The drawing under review shows one solid part. Ordinate dimensions are in mm from its lowest x, y, z. Give positions to 0.01 mm unless a question says otherwise; leave off trailing zeros. Loops run counter-clockwise (first coordinate to the right, second up) from the corner with the lowest first, then second, coordinate; pieces in that order, holes last. Notation, with made-up numbers: M -35.5,58 L -21.5,58 A29 cw -21.5,88 Z; hole C 48.25,49 d3. An arc over 180 degrees is marked long. One line per item, written item: value. Start each with the question number.
Q1. To check wall thickness, follow line 1 along Y through (x, z) = (40.5, 39); line 2 along Y through (x, z) = (42, 30.5) (1 decimal); line 3 along Z through (x, y) = (12.5, 26). State the ranges of each line that lie inside material, in increasing order. Write a range as from..to.
Q2. Mouldability with a two-part tool opening along X and no side actions: class the marked faces 1, 2 and 3 as released by +X, released by -X, zero draft, split by the parting line, or undercut.
Q3. We need section A-A on z = 49. Write out the cut boundary in (x, y) (1 decimal).
Q4. For pin 1 (3 mm diameter, centred on x = 34, z = 46, fed in from +Y); pin 2 (1 mm diameter, centred on x = 44, y = 45.5, fed in from +Z); pin 3 (3 mm diameter, centred on x = 37, z = 49, fed in from -Y) (1 decimal); pin 4 (10 mm diameter, centred on x = 60.5, y = 19, fed in from -Z), all flat-tipped, find the tip position at first contact; note any pin that passes through.
Q5. We need section C-C on y = 62. Write out the cut boundary in (x, z).
Q6. We need section B-B on x = 32. Write out the cut boundary in (y, z), plus the area to 3 significant figures.
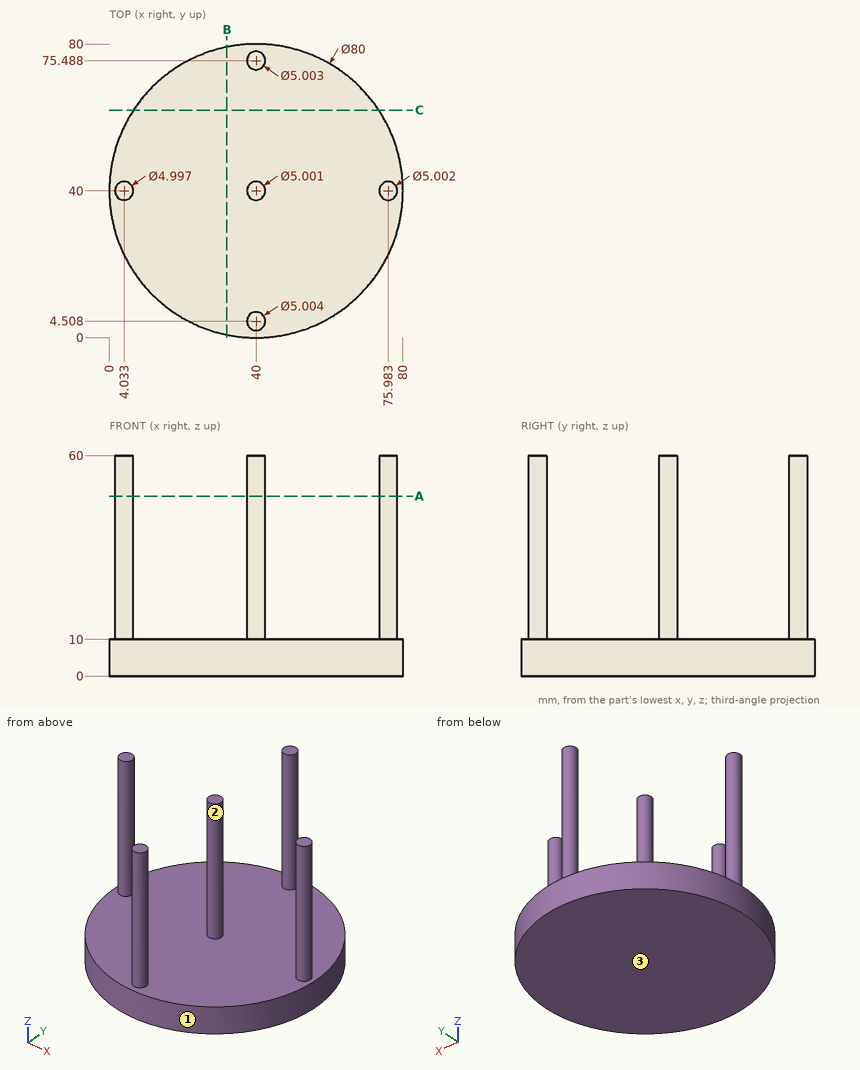
Solved:
1. line 1: 2.06..6.96, 37.55..42.45, 73.04..77.94
1. line 2: 3..6, 38.5..41.5, 74..77
1. line 3: 0..10
2. face 1: split by the parting line
2. face 2: undercut
2. face 3: zero draft
3. outline: C 4,40 d5; C 40,4.5 d5; C 40,40 d5; C 40,75.5 d5; C 76,40 d5
4. pin 1: through
4. pin 2: z = 10
4. pin 3: y = 2.5
4. pin 4: z = 0
5. outline: M 6.59,0 L 73.41,0 L 73.41,10 L 6.59,10 Z
6. outline: M 0.81,0 L 79.19,0 L 79.19,10 L 0.81,10 Z
6. area: 784 mm2
